Could you check a few things on this model? Use its own coordinates, in mm. A direction names the side the tool comes from. Round coordinates to 2 decimals unless told otherwise and drop trailing zeros. Loops run counter-clockwise (first coordinate to the right, second up) from the corner with the lowest first, then second, coordinate; pieces in that order, holes last. Notation, with made-up numbers: (-18, 44.25) -> (8, 44.25) arc R20 cw to (8, 63.25) -> close; hole circle Ø9 at (79, -22). An arc over 180 degrees is marked (long way). One line per item, written item: value.
```python
from build123d import *

# Parameters (mm, degrees)
F0_R     = 1.5875
F1_DEPTH = 2.54


with BuildPart() as f1:
    # F0 (on Top) → F1 (new body)
    with BuildSketch(Plane.XY):
        Polygon((0.193984, 2.904109), (-4.0581, 6.449514), (-2.702028, 1.081909), (-7.387874, -1.866473), (-1.863929, -2.235453), (-0.507857, -7.603057), (1.550056, -2.463495), (7.074001, -2.832475), (2.821917, 0.712929), (4.87983, 5.852492), align=None)
        Circle(F0_R, mode=Mode.SUBTRACT)
    extrude(amount=F1_DEPTH)


solid = f1.part
```
(1) Imagine slicing it at C-C on x = 4. Write out the boundary of the cut face in (y, z).
Results below:
outline: (-2.63, 0) -> (-0.27, 0) -> (-0.27, 2.54) -> (-2.63, 2.54) -> close; (3.66, 0) -> (5.3, 0) -> (5.3, 2.54) -> (3.66, 2.54) -> close
(2) Imagine slicing it at A-A on z = 1.2. Write out the boundary of the cut face in (x, y) (1 decimal).
Results below:
outline: (-7.4, -1.9) -> (-1.9, -2.2) -> (-0.5, -7.6) -> (1.6, -2.5) -> (7.1, -2.8) -> (2.8, 0.7) -> (4.9, 5.9) -> (0.2, 2.9) -> (-4.1, 6.4) -> (-2.7, 1.1) -> close; hole circle Ø3.2 at (0, 0)
(3) Imagine slicing it at B-B on y = 4.5. Write out the boundary of the cut face in (x, z), then the cut area to 3 significant figures.
Results below:
outline: (-3.57, 0) -> (-1.72, 0) -> (-1.72, 2.54) -> (-3.57, 2.54) -> close; (2.73, 0) -> (4.34, 0) -> (4.34, 2.54) -> (2.73, 2.54) -> close
area: 8.77 mm²
(4) We'd pull the mould along X, two halves only. Please class faces 1 (the face through (-1.9, 4.65, 1.25)), 2 (the face through (1, 2, 2.54)), 3 (the face through (-4.66, -2.05, 1.25)): +X half, -X half, draft (parallel to the pull), parting line (faces both ways), or undercut.
Results below:
face 1: undercut
face 2: draft
face 3: -X half
(5) Please list where these lines run through material, in increasing order: L1, parallel to X at y = 4, z = 0.9; L2, parallel to Y at x = 0, z = 1; L3, parallel to Y at x = 3, z = 1.4.
Results below:
L1: x = -3.44 to -1.12, 1.94 to 4.14
L2: y = -6.33 to -1.59, 1.59 to 3.07
L3: y = -2.56 to 0.56, 1.16 to 4.67
(6) On a 3-axis mill with a long thin cutter (end or side, diameter ignored), from which of +Z, -Z, +X, -X, +Y, -Y can I reach the whole of each face in a straight line? I mean faces 4 (the face through (4.978, -1.085, 1.252)), 5 (the face through (4.273, -2.645, 1.252)), 6 (the face through (-5.01, -0.37, 1.25)). Say none if no direction works.
Results below:
face 4: +Z, -Z, +X
face 5: +Z, -Z, -Y
face 6: +Z, -Z, -X
(7) For pin 1 Ø4 at (x, y) = (2, -5) entering from -Z; pin 2 Ø1.5 at (y, z) = (-5.5, 1.5) entering from -X; pin 3 Ø3 at (x, y) = (0, 0) entering from +Z, each with a flat end and sliding along its axis, tell me the tip position at first contact or that it passes through.
Results below:
pin 1: stops at z = 0
pin 2: stops at x = -1.23
pin 3: passes through
(8) Imagine slicing it at D-D on x = 5.5. Write out the boundary of the cut face in (y, z).
Results below:
outline: (-2.73, 0) -> (-1.52, 0) -> (-1.52, 2.54) -> (-2.73, 2.54) -> close
